```python
from build123d import *

# Parameters (mm, degrees)
CROQUIS1_R              = 380
CROQUIS1_R_2            = 18.75
SALIENTE_EXTRUIR1_DEPTH = 10
CROQUIS2_R              = 4
CORTAR_EXTRUIR1_DEPTH   = 538.494186015
REDONDEO1_R             = 5


with BuildPart() as part:
    # Croquis1 → Saliente-Extruir1 (new body)
    with BuildSketch(Plane(origin=(0, 0, 0), x_dir=(1, 0, 0), z_dir=(0, 1, 0))):
        with Locations(Location((0, 0, 0), (0, 0, 270))):
            Circle(CROQUIS1_R)
        with Locations(Location((0, 0, 0), (0, 0, 270))):
            Circle(CROQUIS1_R_2, mode=Mode.SUBTRACT)
    extrude(amount=SALIENTE_EXTRUIR1_DEPTH)

    # Croquis2 → Cortar-Extruir1 (cut, through all)
    with BuildSketch(Plane(origin=(0, 10, 0), x_dir=(1, 0, 0), z_dir=(0, 1, 0))):
        with Locations(Location((-25, -43.301270189, 0), (0, 0, 270))):
            Circle(CROQUIS2_R)
        with Locations(Location((-50, 0, 0), (0, 0, 270))):
            Circle(CROQUIS2_R)
        with Locations(Location((-25, 43.301270189, 0), (0, 0, 270))):
            Circle(CROQUIS2_R)
        with Locations(Location((25, 43.301270189, 0), (0, 0, 270))):
            Circle(CROQUIS2_R)
        with Locations(Location((50, 0, 0), (0, 0, 270))):
            Circle(CROQUIS2_R)
        with Locations(Location((25, -43.301270189, 0), (0, 0, 270))):
            Circle(CROQUIS2_R)
    extrude(amount=-CORTAR_EXTRUIR1_DEPTH, mode=Mode.SUBTRACT)

    # Redondeo1
    redondeo1_edges = [part.edges().sort_by_distance(p)[0] for p in [
        (0, 0, -380),
        (0, 10, -380),
    ]]
    fillet(redondeo1_edges, radius=REDONDEO1_R - 0.0001)  # a hair under: the kernel refuses the full size


solid = part.part
```
Geometry: final body of the model. Coordinates: model frame, mm. Coordinates: 2 decimals unless noted, no trailing zeros. Loops run counter-clockwise (first coordinate to the right, second up) from the corner with the lowest first, then second, coordinate; pieces in that order, holes last. Notation, with made-up numbers: (76.25, -21) -> (127.25, -21) arc R29 cw to (127.25, 18) -> close; hole circle Ø3 at (-16, -8). An arc over 180 degrees is marked (long way). Use a Markdown table: item, result. Add a question column.
(1) Line query: line 1 along X through (y, z) = (6.25, 0); line 2 along X through (y, z) = (3.5, 0); line 3 along Z through (x, y) = (14, 2). Output: solid intervals per line, ascending.
(2) Section query B-B, the plane y = 3.25. Return loops of the section in (x, z), plus the area to 3 significant figures.
(3) Pin query (flat end, axial travel): pin 1 Ø3 at (x, y) = (125.5, 8) entering from -Z; pin 2 Ø13 at (x, z) = (-50, 0) entering from +Y; pin 3 Ø1 at (x, y) = (-236.5, 1.5) entering from -Z; pin 4 Ø6.5 at (x, z) = (25, -43.3) entering from +Y. Return the tip coordinate at first contact, or that it passes through.
(4) Mould query, pull axis Z, two halves, no side actions, for faces 1 (the flat face through (5, 0, 78)), 2 (the cylindrical face through (-11.41, 4.93, -14.88)). Classes: pulls with the +Z half, pulls with the -Z half, needs draft (parallel to the pull), parting line crosses it, or undercut.
Answer:
| question | item | result |
|---|---|---|
| 1 | line 1 | x = -379.84 to -54, -46 to -18.75, 18.75 to 46, 54 to 379.84 |
| 1 | line 2 | x = -379.77 to -54, -46 to -18.75, 18.75 to 46, 54 to 379.77 |
| 1 | line 3 | z = -378.74 to -12.47, 12.47 to 378.74 |
| 2 | outline | circle Ø759.37 at (0, 0); hole circle Ø8 at (-50, 0); hole circle Ø8 at (-25, -43.3); hole circle Ø8 at (-25, 43.3); hole circle Ø37.5 at (0, 0); hole circle Ø8 at (25, -43.3); hole circle Ø8 at (25, 43.3); hole circle Ø8 at (50, 0) |
| 2 | area | 451,000 mm^2 |
| 3 | pin 1 | stops at z = -358.64 |
| 3 | pin 2 | stops at y = 10 |
| 3 | pin 3 | stops at z = -296.3 |
| 3 | pin 4 | passes through |
| 4 | face 1 | needs draft |
| 4 | face 2 | undercut |
